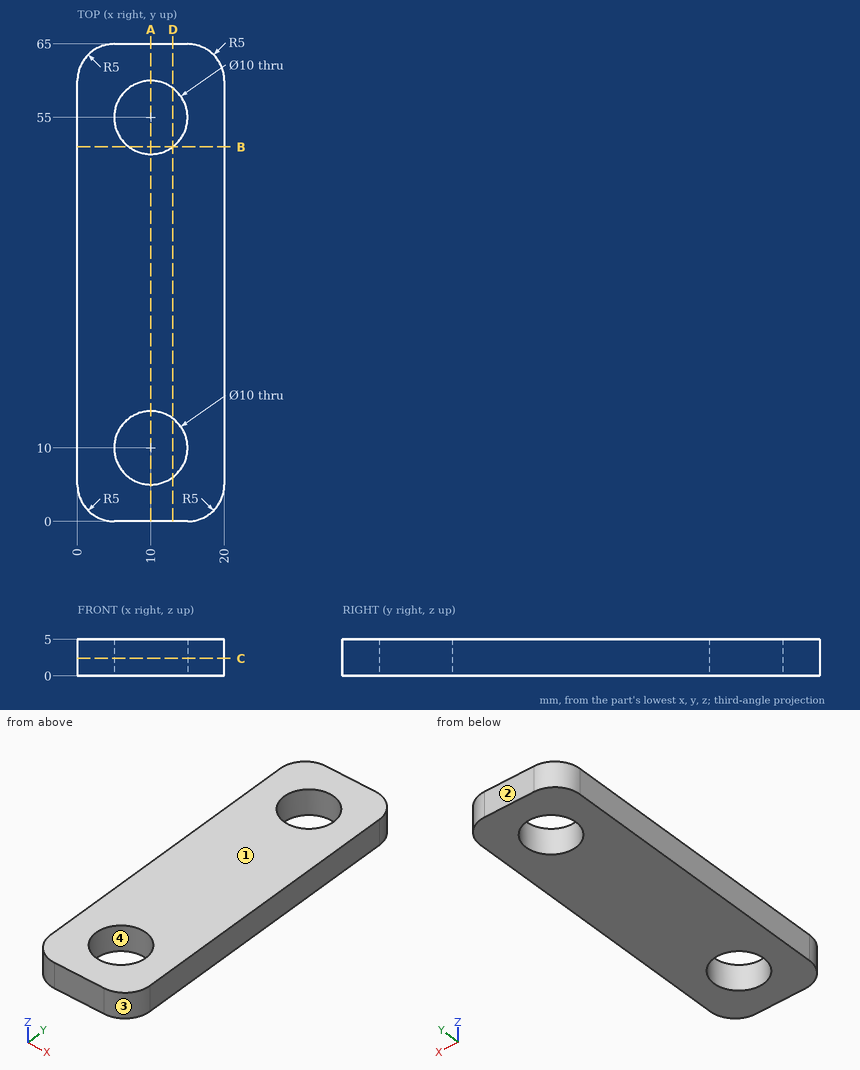
Drawing for the job (mm, zero at the part's lowest x, y, z). Round coordinates to 2 decimals unless told otherwise and drop trailing zeros. Write each loop counter-clockwise with the first axis right and the second up, starting at its lowest first coordinate (ties: lowest second). Pieces come first, ordered by that corner, then holes. Notation, with made-up numbers: (61, 69) - (117, 69) arc R16 ccw to (117, 82) - close; hole circle Ø9 at (14.25, 30.25). An arc over 180 degrees is marked (long way). Return JSON: item names as keys, results as strings. Group by question number.
Item 1: Band-saw the part on D-D on x = 13. List the corners of the cut face in (y, z), plus the area to 3 significant figures.
Item 2: Band-saw the part on B-B on y = 51. List the corners of the cut face in (x, z), plus the area to 3 significant figures.
Item 3: Band-saw the part on A-A on x = 10. List the corners of the cut face in (y, z), plus the area to 3 significant figures.
Item 4: Mould opens along Y. For the marked faces 1, 2, 3 and 4 say: +Y half, -Y half, draft (parallel to the pull), parting line (faces both ways), or undercut.
Item 5: Flat gauge pin, fed straight in: pin 1 Ø8 at (x, y) = (10, 10) entering from +Z. Where does the tip first touch, or does it go through?
Item 6: Band-saw the part on C-C on z = 2.4. List the corners of the cut face in (x, y), plus the area to 3 significant figures.
Item 7: Probe probe 1 along Y at (x, z) = (10, 1.2); probe 2 along Y at (x, z) = (11.25, 1.6); probe 3 along X at (y, z) = (8.5, 4.3). List the from-to ranges inside material, lowest first.
Resolved:
{
 "1": {"outline": "(0, 0) - (6, 0) - (6, 5) - (0, 5) - close; (14, 0) - (51, 0) - (51, 5) - (14, 5) - close; (59, 0) - (65, 0) - (65, 5) - (59, 5) - close", "area": "245 mm²"},
 "2": {"outline": "(0, 0) - (7, 0) - (7, 5) - (0, 5) - close; (13, 0) - (20, 0) - (20, 5) - (13, 5) - close", "area": "70.0 mm²"},
 "3": {"outline": "(0, 0) - (5, 0) - (5, 5) - (0, 5) - close; (15, 0) - (50, 0) - (50, 5) - (15, 5) - close; (60, 0) - (65, 0) - (65, 5) - (60, 5) - close", "area": "225 mm²"},
 "4": {"face 1": "draft", "face 2": "+Y half", "face 3": "-Y half", "face 4": "undercut"},
 "5": {"pin 1": "passes through"},
 "6": {"outline": "(0, 5) arc R5 ccw to (5, 0) - (15, 0) arc R5 ccw to (20, 5) - (20, 60) arc R5 ccw to (15, 65) - (5, 65) arc R5 ccw to (0, 60) - close; hole circle Ø10 at (10, 10); hole circle Ø10 at (10, 55)", "area": "1,120 mm²"},
 "7": {"probe 1": "y = 0 to 5, 15 to 50, 60 to 65", "probe 2": "y = 0 to 5.16, 14.84 to 50.16, 59.84 to 65", "probe 3": "x = 0 to 5.23, 14.77 to 20"}
}
